from build123d import *

# Parameters (mm, degrees)
SKETCH1_R           = 20
BOSS_EXTRUDE1_DEPTH = 10
SKETCH2_W           = 16
SKETCH2_H           = 40
BOSS_EXTRUDE2_DEPTH = 20
SKETCH3_W           = 16
SKETCH3_H           = 22
SKETCH3_R           = 4.75
BOSS_EXTRUDE3_DEPTH = 6
FILLET1_R           = 5
BOSS_EXTRUDE4_START = 10
BOSS_EXTRUDE4_DEPTH = 10


with BuildPart() as part:
    # Sketch1 → Boss-Extrude1 (new body)
    # profile 1 of 2: a face of its own
    with BuildSketch(Plane(origin=(0, 0, 0), x_dir=(1, 0, 0), z_dir=(0, 1, 0))):
        with Locations(Location((0, 0, 0), (0, 0, 270))):
            Circle(SKETCH1_R)
        with BuildLine():
            ThreePointArc((9.191342951, -6.75), (11.691342951, -9.25), (14.191342951, -6.75))
            ThreePointArc((14.191342951, -6.75), (11.691342951, -4.25), (9.191342951, -6.75))
        make_face(mode=Mode.SUBTRACT)
        with BuildLine():
            ThreePointArc((-2.5, -13.5), (0, -16), (2.5, -13.5))
            ThreePointArc((2.5, -13.5), (0, -11), (-2.5, -13.5))
        make_face(mode=Mode.SUBTRACT)
        with BuildLine():
            ThreePointArc((-14.191342951, -6.75), (-11.691342951, -9.25), (-9.191342951, -6.75))
            ThreePointArc((-9.191342951, -6.75), (-11.691342951, -4.25), (-14.191342951, -6.75))
        make_face(mode=Mode.SUBTRACT)
        with BuildLine():
            ThreePointArc((-14.191342951, 6.75), (-11.691342951, 4.25), (-9.191342951, 6.75))
            ThreePointArc((-9.191342951, 6.75), (-11.691342951, 9.25), (-14.191342951, 6.75))
        make_face(mode=Mode.SUBTRACT)
        with BuildLine():
            ThreePointArc((5.5, 0), (0, 5.5), (-5.5, 0))
            ThreePointArc((-5.5, 0), (0, -5.5), (5.5, 0))
        make_face(mode=Mode.SUBTRACT)
        with BuildLine():
            ThreePointArc((-2.5, 13.5), (0, 11), (2.5, 13.5))
            ThreePointArc((2.5, 13.5), (0, 16), (-2.5, 13.5))
        make_face(mode=Mode.SUBTRACT)
        with BuildLine():
            ThreePointArc((9.191342951, 6.75), (11.691342951, 4.25), (14.191342951, 6.75))
            ThreePointArc((14.191342951, 6.75), (11.691342951, 9.25), (9.191342951, 6.75))
        make_face(mode=Mode.SUBTRACT)
    # profile 2 of 2: a face of its own
    with BuildSketch(Plane(origin=(0, 0, 0), x_dir=(1, 0, 0), z_dir=(0, 1, 0))):
        with BuildLine():
            ThreePointArc((-5.5, 0), (0, -5.5), (5.5, 0))
            ThreePointArc((5.5, 0), (0, 5.5), (-5.5, 0))
        make_face()
    extrude(amount=BOSS_EXTRUDE1_DEPTH)

    # Sketch2 → Boss-Extrude2 (add)
    with BuildSketch(Plane(origin=(0, 10, 0), x_dir=(1, 0, 0), z_dir=(0, 1, 0))):
        Rectangle(SKETCH2_W, SKETCH2_H)
    extrude(amount=BOSS_EXTRUDE2_DEPTH)

    # Sketch3 → Boss-Extrude3 (add)
    # profile 1 of 2: a face of its own
    with BuildSketch(Plane(origin=(0, 30, 0), x_dir=(1, 0, 0), z_dir=(0, 1, 0))):
        with Locations((0, -31)):
            Rectangle(SKETCH3_W, SKETCH3_H)
        with Locations(Location((0, -30, 0), (0, 0, 270))):
            Circle(SKETCH3_R, mode=Mode.SUBTRACT)
    # profile 2 of 2: a face of its own
    with BuildSketch(Plane(origin=(0, 30, 0), x_dir=(1, 0, 0), z_dir=(0, 1, 0))):
        with Locations((0, 31)):
            Rectangle(SKETCH3_W, SKETCH3_H)
        with Locations(Location((0, 30, 0), (0, 0, 270))):
            Circle(SKETCH3_R, mode=Mode.SUBTRACT)
    extrude(amount=-BOSS_EXTRUDE3_DEPTH)

    # Fillet1
    fillet1_edges = [part.edges().sort_by_distance(p)[0] for p in [
        (0, 24, 20),
        (0, 24, -20),
    ]]
    fillet(fillet1_edges, radius=FILLET1_R)

    # Sketch4 → Boss-Extrude4 (add)
    with BuildSketch(Plane.XZ.offset(-10).offset(BOSS_EXTRUDE4_START)):
        with BuildLine():
            Line((-8, -18.33030278), (-8, -20))
            Line((-8, -20), (0, -20))
            ThreePointArc((0, -20), (-4.086192874, -19.578126259), (-8, -18.33030278))
        make_face()
        with BuildLine():
            ThreePointArc((8, -18.33030278), (4.086192874, -19.578126259), (0, -20))
            Line((0, -20), (8, -20))
            Line((8, -20), (8, -18.33030278))
        make_face()
        with BuildLine():
            Line((8, 18.33030278), (8, 20))
            Line((8, 20), (0, 20))
            ThreePointArc((0, 20), (4.086192874, 19.578126259), (8, 18.33030278))
        make_face()
        with BuildLine():
            ThreePointArc((-8, 18.33030278), (-4.086192874, 19.578126259), (0, 20))
            Line((0, 20), (-8, 20))
            Line((-8, 20), (-8, 18.33030278))
        make_face()
    extrude(amount=-BOSS_EXTRUDE4_DEPTH)


solid = part.part
Check sheet for the modelled part. Datum: model origin and axes. Units: mm. A direction names the side the tool comes from. Round coordinates to 2 decimals unless told otherwise and drop trailing zeros. Write each loop counter-clockwise with the first axis right and the second up, starting at its lowest first coordinate (ties: lowest second). Pieces come first, ordered by that corner, then holes. Notation, with made-up numbers: (-15, -34.75) - (30, -34.75) arc R23 ccw to (30, -8.75) - close; hole circle Ø4 at (-5, 70.25). An arc over 180 degrees is marked (long way). Return JSON: item names as keys, results as strings.
Q1. Cross-section at A-A (y = 8.5). Record the boundary of the cut face in (x, z), then the cut area to 3 significant figures.
Returned:
{"outline": "(-8, -20) - (8, -20) - (8, -18.33) arc R20 ccw to (8, 18.33) - (8, 20) - (-8, 20) - (-8, 18.33) arc R20 ccw to (-8, -18.33) - close; hole circle Ø5 at (-11.69, -6.75); hole circle Ø5 at (-11.69, 6.75); hole circle Ø5 at (0, -13.5); hole circle Ø5 at (0, 13.5); hole circle Ø5 at (11.69, -6.75); hole circle Ø5 at (11.69, 6.75)", "area": "1,160 mm²"}
Q2. Depth check by flat-ended pin: P1, Ø6, axis at x = 11.69, z = 6.75, coming from the +Y side; P2, Ø15, axis at y = 7.5, z = -13.5, coming from the +X side; P3, Ø4.5, axis at x = 0, z = 13.5, coming from the -Y side. Enter the tip coordinate at first touch or a pass-through.
Returned:
{"P1": "stops at y = 10", "P2": "stops at x = 19.08", "P3": "stops at y = 10"}
Q3. Scan lines: L1, parallel to Z at x = 0, y = 4; L2, parallel to X at y = 2.5, z = -6.75; L3, parallel to X at y = 26.6, z = -30. Record each from-to range of solid material in increasing order. Write a range as from..to.
Returned:
{"L1": "z = -20..-16, -11..11, 16..20", "L2": "x = -18.83..-14.19, -9.19..9.19, 14.19..18.83", "L3": "x = -8..-4.75, 4.75..8"}
Q4. Cross-section at D-D (z = 6.75). Record the boundary of the cut face in (x, y).
Returned:
{"outline": "(-18.83, 0) - (-14.19, 0) - (-14.19, 10) - (-18.83, 10) - close; (-9.19, 0) - (9.19, 0) - (9.19, 10) - (8, 10) - (8, 30) - (-8, 30) - (-8, 10) - (-9.19, 10) - close; (14.19, 0) - (18.83, 0) - (18.83, 10) - (14.19, 10) - close"}
Q5. Cross-section at B-B (z = 30). Record the boundary of the cut face in (x, y).
Returned:
{"outline": "(-8, 24) - (-4.75, 24) - (-4.75, 30) - (-8, 30) - close; (4.75, 24) - (8, 24) - (8, 30) - (4.75, 30) - close"}
Q6. Access from +Z, -Z, +X, -X, +Y, -Y to the whole of each face (thin tool, end or side, straight path). Record for faces 4 (the flat face through (0, 10, -14)), 5 (the flat face through (0, 9, 20)), 6 (the flat face through (0, 9, -20)), 7 (the flat face through (13, 10, 0)).
Returned:
{"face 4": "-Y", "face 5": "+Z, +X, -X, -Y", "face 6": "-Z, +X, -X, -Y", "face 7": "+Z, -Z, +X, +Y"}
Q7. Cross-section at C-C (x = 0). Record the boundary of the cut face in (y, z).
Returned:
{"outline": "(0, -20) - (19, -20) arc R5 cw to (24, -25) - (24, -25.25) - (30, -25.25) - (30, 25.25) - (24, 25.25) - (24, 25) arc R5 cw to (19, 20) - (0, 20) - (0, 16) - (10, 16) - (10, 11) - (0, 11) - (0, -11) - (10, -11) - (10, -16) - (0, -16) - close; (24, -42) - (30, -42) - (30, -34.75) - (24, -34.75) - close; (24, 34.75) - (30, 34.75) - (30, 42) - (24, 42) - close"}
Q8. Draft check along X on faces 1 (the cylindrical face through (0, 22, 21)), 2 (the cylindrical face through (-9.307, 4.93, -7.501)), 3 (the flat face through (-8, 21, 1)). Enter one of: released by +X, released by -X, zero draft, split by the parting line, or undercut.
Returned:
{"face 1": "zero draft", "face 2": "undercut", "face 3": "released by -X"}
